Source: CAD feature listing. Evaluate the final solid. Frame: model axes, mm. A direction names the side the tool comes from. Round coordinates to 2 decimals unless told otherwise and drop trailing zeros. Write each loop counter-clockwise with the first axis right and the second up, starting at its lowest first coordinate (ties: lowest second). Pieces come first, ordered by that corner, then holes. Notation, with made-up numbers: M -24.5,-20 L 7.5,-20 A27 ccw 7.5,12 Z; hole C 40.5,45 d4. An arc over 180 degrees is marked long. Use a Markdown table: item, result.
```python
from build123d import *

# Parameters (mm, degrees)
BOSS_EXTRUDE1_DEPTH = 2.5
SKETCH3_R           = 0.75
BOSS_EXTRUDE2_DEPTH = 1.5
SKETCH4_R           = 0.35
BOSS_EXTRUDE3_DEPTH = 0.7
CHAMFER1_SIZE       = 0.2
CHAMFER2_SIZE       = 0.3
CHAMFER3_SIZE       = 1
SKETCH5_W           = 0.4
SKETCH5_H           = 0.45
BOSS_EXTRUDE4_DEPTH = 4
SKETCH6_R           = 0.740287865
CUT_EXTRUDE1_DEPTH  = 1


with BuildPart() as part:
    # Sketch1 → Boss-Extrude1 (new body, symmetric)
    with BuildSketch(Plane(origin=(0, 0, 0), x_dir=(1, 0, 0), z_dir=(0, 1, 0))):
        Polygon((5, 2.5), (9.3, 2.5), (9.3, -12.7), (-9.3, -12.7), (-9.3, 2.5), (-5, 2.5), (-5, -9.7), (5, -9.7), align=None)
    extrude(amount=BOSS_EXTRUDE1_DEPTH, both=True)

    # Sketch3 → Boss-Extrude2 (add)
    with BuildSketch(Plane.XY.offset(12.7)):
        Circle(SKETCH3_R)
    extrude(amount=BOSS_EXTRUDE2_DEPTH)

    # Sketch4 → Boss-Extrude3 (add)
    with BuildSketch(Plane.XY.offset(12.7)):
        with Locations((8.95, 2)):
            Circle(SKETCH4_R)
    extrude(amount=BOSS_EXTRUDE3_DEPTH)

    # Chamfer1
    chamfer1_edges = [part.edges().sort_by_distance(p)[0] for p in [
        (8.6, 2, 13.4),
    ]]
    chamfer(chamfer1_edges, length=CHAMFER1_SIZE)

    # Chamfer2
    chamfer2_edges = [part.edges().sort_by_distance(p)[0] for p in [
        (-0.75, 0, 14.2),
    ]]
    chamfer(chamfer2_edges, length=CHAMFER2_SIZE)

    # Chamfer3
    chamfer3_edges = [part.edges().sort_by_distance(p)[0] for p in [
        (-7.15, -2.5, -2.5),
        (7.15, -2.5, -2.5),
    ]]
    chamfer(chamfer3_edges, length=CHAMFER3_SIZE)

    # Sketch5 → Boss-Extrude4 (add)
    with BuildSketch(Plane.XY.offset(12.7)):
        with Locations((-7.6, 1.27)):
            Rectangle(SKETCH5_W, SKETCH5_H)
        with Locations((-7.6, -1.27)):
            Rectangle(SKETCH5_W, SKETCH5_H)
        with Locations((-6.1, 0)):
            Rectangle(SKETCH5_W, SKETCH5_H)
        with Locations((7.6, 1.27)):
            Rectangle(SKETCH5_W, SKETCH5_H)
        with Locations((7.6, -1.27)):
            Rectangle(SKETCH5_W, SKETCH5_H)
    extrude(amount=BOSS_EXTRUDE4_DEPTH)

    # Sketch6 → Cut-Extrude1 (cut)
    with BuildSketch(Plane(origin=(-5, 0, 0), x_dir=(0, 0, -1), z_dir=(1, 0, 0))):
        Circle(SKETCH6_R)
    extrude(amount=-CUT_EXTRUDE1_DEPTH, mode=Mode.SUBTRACT)


solid = part.part
```
Q1. Section C-C on y = 0. Return loops of the section in (x, z).
Results are:
| item | result |
|---|---|
| outline | M -9.3,-2.5 L -5,-2.5 L -5,-0.74 L -6,-0.74 L -6,0.74 L -5,0.74 L -5,9.7 L 5,9.7 L 5,-2.5 L 9.3,-2.5 L 9.3,12.7 L 0.75,12.7 L 0.75,13.9 L 0.45,14.2 L -0.45,14.2 L -0.75,13.9 L -0.75,12.7 L -5.9,12.7 L -5.9,16.7 L -6.3,16.7 L -6.3,12.7 L -9.3,12.7 Z |
Q2. Section A-A on z = 0. Return loops of the section in (x, y), plus the area to 3 significant figures.
Results are:
| item | result |
|---|---|
| outline | M -9.3,-2.5 L -5,-2.5 L -5,-0.74 L -6,-0.74 L -6,0.74 L -5,0.74 L -5,2.5 L -9.3,2.5 Z; M 5,-2.5 L 9.3,-2.5 L 9.3,2.5 L 5,2.5 Z |
| area | 41.5 mm^2 |
Q3. Section D-D on y = -1.85. Return loops of the section in (x, z).
Results are:
| item | result |
|---|---|
| outline | M -9.3,-2.15 L -5,-2.15 L -5,9.7 L 5,9.7 L 5,-2.15 L 9.3,-2.15 L 9.3,12.7 L -9.3,12.7 Z |
Q4. Mould query, pull axis X, two halves, no side actions, for faces 4 (the flat face through (-6, 0, 0)), 5 (the flat face through (0, -2.5, 10)), 6 (the flat face through (0, 1, 12.7)), 7 (the flat face through (-9.3, 0, 5)). Classes: +X half, -X half, draft (parallel to the pull), parting line (faces both ways), or undercut.
Results are:
| item | result |
|---|---|
| face 4 | undercut |
| face 5 | draft |
| face 6 | undercut |
| face 7 | -X half |
Q5. Reachability of faces 1 (the flat face through (0, 0, 14.2)), 2 (the cylindrical face through (-0.75, 0.03, 13.29)), 3 (the flat face through (0, 0, 9.7)) from +Z, -Z, +X, -X, +Y, -Y: full face, straight path, thin tool, end or side. Return the list, or none.
Results are:
| item | result |
|---|---|
| face 1 | +Z, +X, +Y, -Y |
| face 2 | +Z |
| face 3 | -Z, +Y, -Y |
Q6. Section B-B on x = 0. Return loops of the section in (y, z), plus the area to 3 significant figures.
Results are:
| item | result |
|---|---|
| outline | M -2.5,9.7 L 2.5,9.7 L 2.5,12.7 L 0.75,12.7 L 0.75,13.9 L 0.45,14.2 L -0.45,14.2 L -0.75,13.9 L -0.75,12.7 L -2.5,12.7 Z |
| area | 17.2 mm^2 |
Q7. Line query: L1, parallel to X at y = -1.1, z = 4.75; L2, parallel to Y at x = -5.5, z = 0; L3, parallel to Z at x = 1.75, y = -1. Output: solid intervals per line, ascending.
Results are:
| item | result |
|---|---|
| L1 | -9.3 to -5, 5 to 9.3 |
| L2 | -2.5 to -0.74, 0.74 to 2.5 |
| L3 | 9.7 to 12.7 |
